The model under review builds one solid part; all positions refer to its coordinate system, in mm. A direction names the side the tool comes from. Coordinates: 2 decimals unless noted, no trailing zeros. Write each loop counter-clockwise with the first axis right and the second up, starting at its lowest first coordinate (ties: lowest second). Pieces come first, ordered by that corner, then holes. Notation, with made-up numbers: (-19, -5.75) - (29, -5.75) arc R21 cw to (29, 20.25) - close; hole circle Ø6 at (43.25, -1.5). An arc over 180 degrees is marked (long way). Return JSON: item names as keys, results as strings. Group by question number.
(1) We need section C-C on y = 12. State the section outline as (x, z) points, then the cut area to 3 significant figures.
(2) We need section B-B on x = 0. State the section outline as (y, z) points.
(3) Tool access review of faces 1 (the face through (0, 25, 10)), 2 (the face through (0, 0, -11)): name each direction out of +Z, -Z, +X, -X, +Y, -Y from which nothing blocks a thin tool from reaching the whole face with its end or side.
(4) Draft analysis for pull direction X (two halves, no side actions). For faces 3 (the face through (0, 50, -11)), 4 (the face through (-23.846, 24.65, -7.509)), 5 (the face through (10, 25, 0)), state which applies: released by +X, released by -X, zero draft, split by the parting line, or undercut.
(5) We need section A-A on z = 0. State the section outline as (x, y) points, then the cut area to 3 significant figures.
(6) We need section D-D on x = -19. State the section outline as (y, z) points.
(7) For pin 1 Ø1.5 at (x, y) = (6.5, 18) entering from +Z; pin 2 Ø2 at (y, z) = (7, 9.5) entering from -X; pin 3 Ø6 at (x, y) = (-15, 14.5) entering from +Z, all flat-tipped, find the tip position at first contact; note any pin that passes through.
(8) To check wall thickness, follow L1, parallel to Z at x = 0.5, y = 29.5 (3 decimals); L2, parallel to X at y = 36, z = 4; L3, parallel to X at y = 8, z = 6.5. State the ranges of each line that lie inside material, in increasing order. Write a range as from..to.
Autodesk Inventor part; units mm, degrees
ref_plane "YZ Plane" through (0, 0, 0) normal (1, 0, 0) x (0, 1, 0)
ref_plane "XZ Plane" through (0, 0, 0) normal (0, 1, 0) x (-1, 0, 0)
ref_plane "XY Plane" through (0, 0, 0) normal (0, 0, 1) x (1, 0, 0)
sketch "Sketch1" plane through (0, 0, 0) normal (0, 1, 0) x (-1, 0, 0)
  circle A0 centre (0, 0) radius 25
  line L0 (0, 0) -> (0, 10)
  line L1 (0, 10) -> (10, 10)
  line L2 (10, 10) -> (-10, 10)
  line L3 (-10, 10) -> (-10, -10)
  line L4 (-10, -10) -> (10, -10)
  line L5 (10, -10) -> (10, 10)
  dimension "d0" = 50
  dimension "d1" = 10
  dimension "d2" = 10
  dimension "d3" = 20
  dimension "d4" = 20
extrude "Extrusion1" add sketch "Sketch1" along normal blind 50
properties part number "base"
Ans:
{
 "1": {"outline": "circle Ø50 at (0, 0); hole (-10, -10) - (10, -10) - (10, 10) - (-10, 10) - close", "area": "1,560 mm²"},
 "2": {"outline": "(0, -25) - (50, -25) - (50, -10) - (0, -10) - close; (0, 10) - (50, 10) - (50, 25) - (0, 25) - close"},
 "3": {"face 1": "+Y, -Y", "face 2": "+Z, -Z, +X, -X, -Y"},
 "4": {"face 3": "zero draft", "face 4": "split by the parting line", "face 5": "undercut"},
 "5": {"outline": "(-25, 0) - (-10, 0) - (-10, 50) - (-25, 50) - close; (10, 0) - (25, 0) - (25, 50) - (10, 50) - close", "area": "1,500 mm²"},
 "6": {"outline": "(0, -16.25) - (50, -16.25) - (50, 16.25) - (0, 16.25) - close"},
 "7": {"pin 1": "z = 24.33", "pin 2": "x = -23.51", "pin 3": "z = 21.93"},
 "8": {"L1": "-24.995..-10, 10..24.995", "L2": "-24.68..-10, 10..24.68", "L3": "-24.14..-10, 10..24.14"}
}
